Check sheet for the modelled part. Datum: model origin and axes. Units: mm. A direction names the side the tool comes from. Round coordinates to 2 decimals unless told otherwise and drop trailing zeros. Write each loop counter-clockwise with the first axis right and the second up, starting at its lowest first coordinate (ties: lowest second). Pieces come first, ordered by that corner, then holes. Notation, with made-up numbers: (84, -13.75) -> (138, -13.75) arc R20 cw to (138, 17.25) -> close; hole circle Ø7 at (48, 48.5). An arc over 180 degrees is marked (long way). Write item = value, one per line.
from build123d import *

# Parameters (mm, degrees)
SKETCH_1_W                = 56
SKETCH_1_H                = 56
EXTRUDE_1_DEPTH           = 103
SKETCH_2_W                = 9
SKETCH_2_H                = 9
CUT_EXTRUDE_1_DEPTH       = 99.5
HOLE_WIZARD_5_0_5_1_D     = 5
HOLE_WIZARD_5_0_5_1_DEPTH = 10
HOLE_WIZARD_5_0_5_1_TIP   = 1.502151548
FILLET_2_R                = 5
SKETCH_5_R                = 19
EXTRUDE_2_DEPTH           = 1.5
SKETCH_6_R                = 11
CUT_EXTRUDE_2_DEPTH       = 1
SKETCH_7_R                = 4
EXTRUDE_3_DEPTH           = 20
FILLET_3_R                = 2
SKETCH_8_R                = 26
EXTRUDE_4_DEPTH           = 1.5
CHAMFER_1_SIZE2           = 5.598076211
CHAMFER_1_SIZE            = 1.5


with BuildPart() as part:
    # 草图1 → 凸台-拉伸1 (new body)
    with BuildSketch(Plane.XY):
        with Locations((28, 28)):
            Rectangle(SKETCH_1_W, SKETCH_1_H)
    extrude(amount=EXTRUDE_1_DEPTH)

    # 草图2 → 切除-拉伸1 (cut)
    with BuildSketch(Plane(origin=(0, 0, 0), x_dir=(-1, 0, 0), z_dir=(0, 0, -1))):
        with Locations((-51.5, 4.5)):
            Rectangle(SKETCH_2_W, SKETCH_2_H)
        with Locations((-51.5, 51.5)):
            Rectangle(SKETCH_2_W, SKETCH_2_H)
        with Locations((-4.5, 51.5)):
            Rectangle(SKETCH_2_W, SKETCH_2_H)
        with Locations((-4.5, 4.5)):
            Rectangle(SKETCH_2_W, SKETCH_2_H)
    extrude(amount=-CUT_EXTRUDE_1_DEPTH, mode=Mode.SUBTRACT)

    # Ø5.0 (5) 直径孔1
    with Locations(Plane.XY.offset(103)):
        with Locations((4.5, 51.5), (51.5, 51.5), (51.5, 4.5), (4.5, 4.5)):
            Hole(HOLE_WIZARD_5_0_5_1_D / 2, depth=HOLE_WIZARD_5_0_5_1_DEPTH)
            with Locations((0, 0, -(HOLE_WIZARD_5_0_5_1_DEPTH + HOLE_WIZARD_5_0_5_1_TIP / 2))):  # 118° drill point
                Cone(0, HOLE_WIZARD_5_0_5_1_D / 2, HOLE_WIZARD_5_0_5_1_TIP, mode=Mode.SUBTRACT)

    # 圆角2
    fillet_2_edges = [part.edges().sort_by_distance(p)[0] for p in [
        (47, 9, 49.75),
        (47, 47, 49.75),
        (9, 47, 49.75),
        (9, 9, 49.75),
    ]]
    fillet(fillet_2_edges, radius=FILLET_2_R)

    # 草图5 → 凸台-拉伸2 (add)
    with BuildSketch(Plane.XY.offset(103)):
        with Locations(Location((28, 28, 0), (0, 0, 180))):
            Circle(SKETCH_5_R)
    extrude(amount=EXTRUDE_2_DEPTH)

    # 草图6 → 切除-拉伸2 (cut)
    with BuildSketch(Plane.XY.offset(104.5)):
        with Locations((28, 28)):
            Circle(SKETCH_6_R)
    extrude(amount=-CUT_EXTRUDE_2_DEPTH, mode=Mode.SUBTRACT)

    # 草图7 → 凸台-拉伸3 (add)
    with BuildSketch(Plane.XY.offset(103.5)):
        with Locations((28, 28)):
            Circle(SKETCH_7_R)
    extrude(amount=EXTRUDE_3_DEPTH)

    # 圆角3
    fillet_3_edges = [part.edges().sort_by_distance(p)[0] for p in [
        (56, 9, 49.75),
        (47, 0, 49.75),
        (56, 47, 49.75),
        (47, 56, 49.75),
        (0, 47, 49.75),
        (9, 56, 49.75),
        (0, 9, 49.75),
        (9, 0, 49.75),
        (0, 56, 101.25),
        (56, 56, 101.25),
        (56, 0, 101.25),
        (0, 0, 101.25),
    ]]
    fillet(fillet_3_edges, radius=FILLET_3_R)

    # 草图8 → 凸台-拉伸4 (add)
    with BuildSketch(Plane(origin=(0, 0, 0), x_dir=(-1, 0, 0), z_dir=(0, 0, -1))):
        with Locations((-28, 28)):
            Circle(SKETCH_8_R)
    extrude(amount=EXTRUDE_4_DEPTH)

    # 倒角1
    chamfer_1_edges = [part.edges().sort_by_distance(p)[0] for p in [
        (54, 28, -1.5),
    ]]
    chamfer_1_side = [part.faces().sort_by_distance(p)[0] for p in [
        (54, 28, -1.47),
    ]]
    chamfer(chamfer_1_edges, length=CHAMFER_1_SIZE - 0.0001, length2=CHAMFER_1_SIZE2 - 0.0001, reference=chamfer_1_side[0])  # a hair under: the kernel refuses the full size


solid = part.part
(1) Go/stop test with flat-tipped pins: P1, Ø4.5, axis at x = 51.5, y = 4.5, coming from the +Z side; P2, Ø1, axis at y = 2.5, z = 67, coming from the -X side; P3, Ø1, axis at x = 53, z = 45.5, coming from the -Y side; P4, Ø1, axis at y = 2.5, z = 40, coming from the +X side. Record where each tip stops, or that it passes through.
Worked answers:
P1 = through
P2 = 9
P3 = 9
P4 = 47
(2) Material ranges on L1, parallel to Y at x = 28, z = 104.35; L2, parallel to X at y = 51, z = 100; L3, parallel to X at y = 7.5, z = 80.5, recorded low to high. Write a range as [from, to].
Worked answers:
L1 = [9, 17], [24, 32], [39, 47]
L2 = [0, 2.05], [6.95, 49.05], [53.95, 56]
L3 = [7.57, 48.43]
(3) Sectioned sample at C-C on z = 89. Enter the section's corners in (x, y).
Worked answers:
outline = (0, 11) arc R2 ccw to (2, 9) -> (4, 9) arc R5 cw to (9, 4) -> (9, 2) arc R2 ccw to (11, 0) -> (45, 0) arc R2 ccw to (47, 2) -> (47, 4) arc R5 cw to (52, 9) -> (54, 9) arc R2 ccw to (56, 11) -> (56, 45) arc R2 ccw to (54, 47) -> (52, 47) arc R5 cw to (47, 52) -> (47, 54) arc R2 ccw to (45, 56) -> (11, 56) arc R2 ccw to (9, 54) -> (9, 52) arc R5 cw to (4, 47) -> (2, 47) arc R2 ccw to (0, 45) -> close
(4) Access from +Z, -Z, +X, -X, +Y, -Y to the whole of each face (thin tool, end or side, straight path). Record for faces 4 (the flat face through (54.2, 4.4, 99.5)), 5 (the cylindrical face through (7, 8, 50)), 6 (the flat face through (28, 23, 103.5)).
Worked answers:
face_4 = -Z, +X, -Y
face_5 = -Z, -X, -Y
face_6 = +Z
(5) Release check for a two-part mould opening along Y. For faces 1 (the flat face through (3, 2, 99.5)), 2 (the cylindrical face through (49.19, 3.54, 101.23)), 3 (the flat face through (33, 56, 51)) record: pulls with the +Y half, pulls with the -Y half, needs draft (parallel to the pull), parting line crosses it, or undercut.
Worked answers:
face_1 = needs draft
face_2 = undercut
face_3 = pulls with the +Y half
